```python
from build123d import *

# Parameters (mm, degrees)
SKETCH1_R           = 25.4
BOSS_EXTRUDE2_DEPTH = 7.62
CUT_EXTRUDE2_DEPTH  = 47.498
SKETCH1_5_R         = 1.27
CUT_EXTRUDE5_DEPTH  = 61.214
FILLET3_R           = 1.27
FILLET4_R           = 1.27
SKETCH9_R           = 24.13
CUT_EXTRUDE7_DEPTH  = 5.08


with BuildPart() as part:
    # Sketch1 → Boss-Extrude2 (new body)
    with BuildSketch(Plane(origin=(0, 0, 0), x_dir=(1, 0, 0), z_dir=(0, 1, 0))):
        with Locations(Location((0, 0, 0), (0, 0, 90))):
            Circle(SKETCH1_R)
    extrude(amount=BOSS_EXTRUDE2_DEPTH)

    # Sketch1_4 → Cut-Extrude2 (cut)
    with BuildSketch(Plane(origin=(0, 0, 0), x_dir=(1, 0, 0), z_dir=(0, 1, 0))):
        with BuildLine():
            add(Edge.make_bspline(
                [(-3.273780401, 3.901539579), (-0.461582665, 6.261253705), (-7.342126917, 20.172327916)],
                knots=[0.500000001, 0.500000001, 0.500000001, 1, 1, 1], degree=2))
            ThreePointArc((-7.342126917, 20.172327916), (-13.79868497, 16.444632387), (-18.590917969, 10.733471494))
            add(Edge.make_bspline(
                [(-18.590917969, 10.733471494), (-6.085978149, 1.541825443), (-3.273780401, 3.901539579)],
                knots=[0, 0, 0, 0.500000001, 0.500000001, 0.500000001], degree=2))
        make_face()
        with BuildLine():
            add(Edge.make_bspline(
                [(1.741942169, 4.785946791), (5.19161341, 3.530369129), (13.79868497, 16.444632387)],
                knots=[0.5, 0.5, 0.5, 1, 1, 1], degree=2))
            ThreePointArc((13.79868497, 16.444632387), (7.342126917, 20.172327916), (0, 21.466942988))
            add(Edge.make_bspline(
                [(0, 21.466942988), (-1.707729067, 6.041524451), (1.741942169, 4.785946791)],
                knots=[0, 0, 0, 0.5, 0.5, 0.5], degree=2))
        make_face()
        with BuildLine():
            ThreePointArc((21.140811888, -3.72769553), (21.385254789, -1.870967361), (21.466942988, 0))
            ThreePointArc((21.466942988, 0), (20.735474643, 5.556053685), (18.590917969, 10.733471494))
            add(Edge.make_bspline(
                [(18.590917969, 10.733471494), (4.378249044, 4.499698948), (5.015722593, 0.884407188)],
                knots=[0, 0, 0, 0.500000002, 0.500000002, 0.500000002], degree=2))
            add(Edge.make_bspline(
                [(5.015722593, 0.884407188), (5.653196136, -2.73088454), (21.140811888, -3.72769553)],
                knots=[0.500000002, 0.500000002, 0.500000002, 1, 1, 1], degree=2))
        make_face()
        with BuildLine():
            ThreePointArc((7.342126917, -20.172327916), (13.79868497, -16.444632387), (18.590917969, -10.733471494))
            add(Edge.make_bspline(
                [(18.590917969, -10.733471494), (6.085978062, -1.54182538), (3.273780362, -3.901539612)],
                knots=[0, 0, 0, 0.500000005, 0.500000005, 0.500000005], degree=2))
            add(Edge.make_bspline(
                [(3.273780362, -3.901539612), (0.461582713, -6.261253801), (7.342126917, -20.172327916)],
                knots=[0.500000005, 0.500000005, 0.500000005, 1, 1, 1], degree=2))
        make_face()
        with BuildLine():
            ThreePointArc((-13.79868497, -16.444632387), (-7.342126917, -20.172327916), (0, -21.466942988))
            add(Edge.make_bspline(
                [(0, -21.466942988), (1.707729058, -6.041524539), (-1.741942129, -4.785946805)],
                knots=[0, 0, 0, 0.499999997, 0.499999997, 0.499999997], degree=2))
            add(Edge.make_bspline(
                [(-1.741942129, -4.785946805), (-5.191613361, -3.530369055), (-13.79868497, -16.444632387)],
                knots=[0.499999997, 0.499999997, 0.499999997, 1, 1, 1], degree=2))
        make_face()
        with BuildLine():
            add(Edge.make_bspline(
                [(-18.590917969, -10.733471494), (-4.378249044, -4.499698948), (-5.015722593, -0.884407188)],
                knots=[0, 0, 0, 0.500000002, 0.500000002, 0.500000002], degree=2))
            add(Edge.make_bspline(
                [(-5.015722593, -0.884407188), (-5.653196136, 2.73088454), (-21.140811888, 3.72769553)],
                knots=[0.500000002, 0.500000002, 0.500000002, 1, 1, 1], degree=2))
            ThreePointArc((-21.140811888, 3.72769553), (-21.140811888, -3.72769553), (-18.590917969, -10.733471494))
        make_face()
    extrude(amount=CUT_EXTRUDE2_DEPTH, mode=Mode.SUBTRACT)

    # Sketch1_5 → Cut-Extrude5 (cut)
    with BuildSketch(Plane(origin=(0, 0, 0), x_dir=(1, 0, 0), z_dir=(0, 1, 0))):
        with Locations(Location((0, 0, 0), (0, 0, 90))):
            Circle(SKETCH1_5_R)
    extrude(amount=CUT_EXTRUDE5_DEPTH, mode=Mode.SUBTRACT)

    # Fillet3
    fillet3_edges = [part.edges().sort_by_distance(p)[0] for p in [
        (0, 0, 25.4),
    ]]
    fillet(fillet3_edges, radius=FILLET3_R)

    # Fillet4
    fillet4_edges = [part.edges().sort_by_distance(p)[0] for p in [
        (0, 7.62, 25.4),
    ]]
    fillet(fillet4_edges, radius=FILLET4_R)

    # Sketch9 → Cut-Extrude7 (cut)
    with BuildSketch(Plane(origin=(0, 7.62, 0), x_dir=(1, 0, 0), z_dir=(0, 1, 0))):
        with Locations(Location((0, 0, 0), (0, 0, 270))):
            Circle(SKETCH9_R)
    extrude(amount=-CUT_EXTRUDE7_DEPTH, mode=Mode.SUBTRACT)


solid = part.part
```
Geometry check sheet. Reference: the model listing, model coordinates, mm. A direction names the side the tool comes from. Round coordinates to 2 decimals unless told otherwise and drop trailing zeros. Loops run counter-clockwise (first coordinate to the right, second up) from the corner with the lowest first, then second, coordinate; pieces in that order, holes last. Notation, with made-up numbers: M -14.5,0 L 44.5,0 A31 cw 44.5,24 Z; hole C 31,7.25 d9. An arc over 180 degrees is marked long. Return JSON: item names as keys, results as strings. Group by question number.
(1) Go/stop test with flat-tipped pins: pin 1 (24 mm diameter, centred on x = -6, z = 9.5, fed in from +Y); pin 2 (2 mm diameter, centred on y = 4, z = -15, fed in from +X); pin 3 (2 mm diameter, centred on x = 11.5, y = 1, fed in from +Z). Record where each tip stops, or that it passes through.
(2) Set-up check for faces 1 (the face through (0, 2.54, 5)), 2 (the face through (13.72, 1.25, 16.51)): record each of +Z, -Z, +X, -X, +Y, -Y from which the full face is reachable in a straight line by a thin tool's end or side.
(3) Section check B-B, the plane y = 4.5. Enter the section's corners in (x, z), and give its area (3 significant figures).
(4) Scan lines: line 1 along X through (y, z) = (4.55, 0); line 2 along X through (y, z) = (1, 0); line 3 along Y through (x, z) = (-3.5, -16). Record each from-to range of solid material in increasing order. Write a range as [from, to].
(5) Mould release check, pull along X, two halves, no side actions. Record for faces 3 (the face through (-13.72, 1.25, -16.51)), 4 (the face through (15.456, 3.774, 20.157)), 5 (the face through (0, 0, -5)): pulls with the +X half, pulls with the -X half, needs draft (parallel to the pull), parting line crosses it, or undercut.
(6) Section check A-A, the plane z = 19.5. Give the number of separate pieces and of enclosed holes in the cut face, and give its area (3 significant figures).
Data:
{
 "1": {"pin 1": "y = 2.54", "pin 2": "x = 21.19", "pin 3": "z = 23.12"},
 "2": {"face 1": "+Y", "face 2": "+Y, -Y"},
 "3": {"outline": "C 0,0 d50.8; hole C 0,0 d48.26", "area": "198 mm²"},
 "4": {"line 1": "[-25.4, -24.13], [24.13, 25.4]", "line 2": "[-25.37, -21.47], [-5.42, -1.27], [1.27, 5.42], [21.47, 25.37]", "line 3": "[0, 2.54]"},
 "5": {"face 3": "undercut", "face 4": "parting line crosses it", "face 5": "needs draft"},
 "6": {"separate pieces": "3", "enclosed holes": "0", "area": "73.1 mm²"}
}
